Read the model definition and answer for the solid it produces. Units are mm, in the model's axes. Round coordinates to 2 decimals unless told otherwise and drop trailing zeros. Write each loop counter-clockwise with the first axis right and the second up, starting at its lowest first coordinate (ties: lowest second). Pieces come first, ordered by that corner, then holes.
Solid Edge part; units mm, degrees
sketch "Sketch1" plane through (0, 0, 12.0462) normal (0, 0, 1) x (1, 0, 0)
  circle A0 centre (0, 0) radius 180
extrude "ProtrusioneEstrusa_1" add sketch "Sketch1" along normal blind 15
sketch "Sketch2" plane through (0, 0, 27.0462) normal (0, 0, 1) x (0, 1, 0)
  arc A0 (6.631, -7.4853) -> (3.1669, -9.4853) centre (0, 0) cw
  line L0 (3.1669, -9.4853) -> (2.1409, -7.7082)
  arc A1 (2.1409, -7.7082) -> (-2.1409, -7.7082) centre (0, 0) cw
  line L1 (-2.1409, -7.7082) -> (-3.1669, -9.4853)
  arc A2 (-3.1669, -9.4853) -> (-6.631, -7.4853) centre (0, 0) cw
  line L2 (-6.631, -7.4853) -> (-5.605, -5.7082)
  arc A3 (-5.605, -5.7082) -> (-7.746, -2) centre (0, 0) cw
  line L3 (-7.746, -2) -> (-9.798, -2)
  arc A4 (-9.798, -2) -> (-9.798, 2) centre (0, 0) cw
  line L4 (-9.798, 2) -> (-7.746, 2)
  arc A5 (-7.746, 2) -> (-5.605, 5.7082) centre (0, 0) cw
  line L5 (-5.605, 5.7082) -> (-6.631, 7.4853)
  arc A6 (-6.631, 7.4853) -> (-3.1669, 9.4853) centre (0, 0) cw
  line L6 (-3.1669, 9.4853) -> (-2.1409, 7.7082)
  arc A7 (-2.1409, 7.7082) -> (2.1409, 7.7082) centre (0, 0) cw
  line L7 (2.1409, 7.7082) -> (3.1669, 9.4853)
  arc A8 (3.1669, 9.4853) -> (6.631, 7.4853) centre (0, 0) cw
  line L8 (6.631, 7.4853) -> (5.605, 5.7082)
  arc A9 (5.605, 5.7082) -> (7.746, 2) centre (0, 0) cw
  line L9 (7.746, 2) -> (9.798, 2)
  arc A10 (9.798, 2) -> (9.798, -2) centre (0, 0) cw
  line L10 (9.798, -2) -> (7.746, -2)
  arc A11 (7.746, -2) -> (5.605, -5.7082) centre (0, 0) cw
  line L11 (5.605, -5.7082) -> (6.631, -7.4853)
extrude "Cutout1" cut sketch "Sketch2" against normal through all
sketch "Sketch3" plane through (0, 0, 27.0462) normal (0, 0, 1) x (-1, 0, 0)
  arc A0 (-169.7056, 60) -> (-180, 0) centre (-137.739, 23.6323) ccw
extrude "Protrusion1" add sketch "Sketch3" against normal up to vertex (15 mm away) material side at (185.4122, -31.8117, 27.0462)
properties material "Policarbonato"
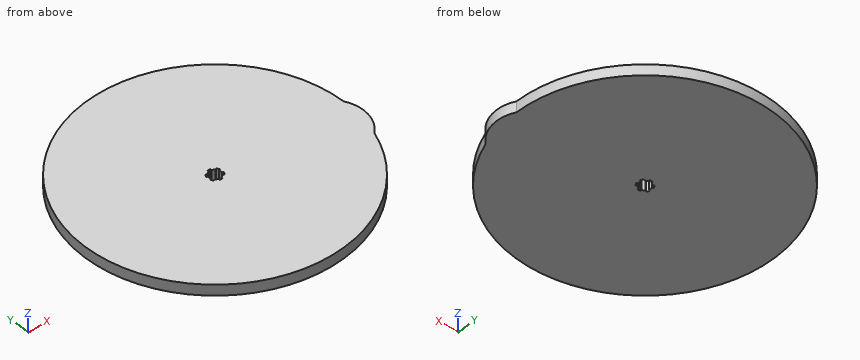
Q1. Straight lines are drawn through the part: probe 1 along X at (y, z) = (2, 18.75); probe 2 along X at (y, z) = (-93, 20); probe 3 along Y at (x, z) = (147.5, 18). For each, find the intervals that lie inside material, in ascending order.
Verdict:
probe 1: x = -179.99 to -7.75, 7.75 to 179.99
probe 2: x = -154.11 to 154.11
probe 3: y = -103.17 to 103.17
Q2. Flat-ended cylindrical pins translate along their axes: pin 1 Ø5 at (y, z) = (64, 23) entering from +X; pin 2 Ø1.5 at (y, z) = (64.5, 23) entering from +X; pin 3 Ø2 at (x, z) = (115, 22.5) entering from -Y. Find the tip coordinate at first contact, or state that the pin passes through.
Verdict:
pin 1: stops at x = 169.17
pin 2: stops at x = 168.33
pin 3: stops at y = -139.3
Q3. Section C-C (x = -57) is taken. Determine the outline of the cut face in (y, z).
Verdict:
outline: (-170.74, 12.05) - (170.74, 12.05) - (170.74, 27.05) - (-170.74, 27.05) - close
Q4. Section B-B (y = -92) is taken. Determine the outline of the cut face in (x, z), then the cut area to 3 significant figures.
Verdict:
outline: (-154.71, 12.05) - (154.71, 12.05) - (154.71, 27.05) - (-154.71, 27.05) - close
area: 4,640 mm2
Q5. Section A-A (z = 19) is taken. Determine the outline of the cut face in (x, y).
Verdict:
outline: (169.71, -60) arc R48.42 ccw to (180, 0) arc R180 ccw (long way) to start; hole (-9.49, -3.17) arc R10 ccw to (-7.49, -6.63) - (-5.71, -5.61) arc R8 ccw to (-2, -7.75) - (-2, -9.8) arc R10 ccw to (2, -9.8) - (2, -7.75) arc R8 ccw to (5.71, -5.61) - (7.49, -6.63) arc R10 ccw to (9.49, -3.17) - (7.71, -2.14) arc R8 ccw to (7.71, 2.14) - (9.49, 3.17) arc R10 ccw to (7.49, 6.63) - (5.71, 5.61) arc R8 ccw to (2, 7.75) - (2, 9.8) arc R10 ccw to (-2, 9.8) - (-2, 7.75) arc R8 ccw to (-5.71, 5.61) - (-7.49, 6.63) arc R10 ccw to (-9.49, 3.17) - (-7.71, 2.14) arc R8 ccw to (-7.71, -2.14) - close
